from build123d import *

# Parameters (mm, degrees)
ESBO_O1_R                = 0.5
RESSALTO_EXTRUS_O1_DEPTH = 5


with BuildPart() as part:
    # Esboço1 → Ressalto-extrusão1 (new body)
    with BuildSketch(Plane.XZ.offset(5)):
        with BuildLine():
            ThreePointArc((0.88816946, -1.287165167), (0.853822869, -1.148958648), (0.919306865, -1.022496889))
            ThreePointArc((0.919306865, -1.022496889), (0.972271824, -0.972271824), (1.022496889, -0.919306865))
            ThreePointArc((1.022496889, -0.919306865), (1.148958648, -0.853822869), (1.287165167, -0.88816946))
            add(Edge.make_bspline(
                [(1.287165167, -0.88816946), (1.383791359, -0.954882813), (1.556408334, -1.073982269), (1.549215881, -1.068804746), (1.613247697, -1.099886307), (1.689593731, -1.118505632), (1.818337157, -1.137704346), (2.003981613, -1.135749512), (2.169907523, -1.103671613), (2.254570833, -1.080236252)],
                knots=[0.030903034, 0.030903034, 0.030903034, 0.030903034, 0.091208758, 0.151514483, 0.272125931, 0.39273738, 0.513348828, 0.754571725, 0.995794622, 0.995794622, 0.995794622, 0.995794622], degree=3))
            ThreePointArc((2.254570833, -1.080236252), (2.309698831, -0.956708581), (2.358064704, -0.830379945))
            add(Edge.make_bspline(
                [(1.538193866, -0.28213257), (1.653692366, -0.303284141), (1.859967032, -0.341126742), (1.851220139, -0.339701972), (1.918475453, -0.36300132), (1.985626101, -0.403820267), (2.090236992, -0.481280077), (2.220125169, -0.613932807), (2.314770006, -0.753942643), (2.358064704, -0.830379945)],
                knots=[0.030903034, 0.030903034, 0.030903034, 0.030903034, 0.091208758, 0.151514483, 0.272125931, 0.39273738, 0.513348828, 0.754571725, 0.995794622, 0.995794622, 0.995794622, 0.995794622], degree=3))
            ThreePointArc((1.538193866, -0.28213257), (1.416180392, -0.208692511), (1.373062602, -0.072966366))
            ThreePointArc((1.373062602, -0.072966366), (1.375, 0), (1.373062602, 0.072966366))
            ThreePointArc((1.373062602, 0.072966366), (1.416180392, 0.208692511), (1.538193866, 0.28213257))
            add(Edge.make_bspline(
                [(1.538193866, 0.28213257), (1.653692366, 0.303284141), (1.859967032, 0.341126742), (1.851220139, 0.339701972), (1.918475453, 0.36300132), (1.985626101, 0.403820267), (2.090236992, 0.481280077), (2.220125169, 0.613932807), (2.314770006, 0.753942643), (2.358064704, 0.830379945)],
                knots=[0.030903034, 0.030903034, 0.030903034, 0.030903034, 0.091208758, 0.151514483, 0.272125931, 0.39273738, 0.513348828, 0.754571725, 0.995794622, 0.995794622, 0.995794622, 0.995794622], degree=3))
            ThreePointArc((2.358064704, 0.830379945), (2.309698831, 0.956708581), (2.254570833, 1.080236252))
            add(Edge.make_bspline(
                [(1.287165167, 0.88816946), (1.383791359, 0.954882813), (1.556408334, 1.073982269), (1.549215881, 1.068804746), (1.613247697, 1.099886307), (1.689593731, 1.118505632), (1.818337157, 1.137704346), (2.003981613, 1.135749512), (2.169907523, 1.103671613), (2.254570833, 1.080236252)],
                knots=[0.030903034, 0.030903034, 0.030903034, 0.030903034, 0.091208758, 0.151514483, 0.272125931, 0.39273738, 0.513348828, 0.754571725, 0.995794622, 0.995794622, 0.995794622, 0.995794622], degree=3))
            ThreePointArc((1.287165167, 0.88816946), (1.148958648, 0.853822869), (1.022496889, 0.919306865))
            ThreePointArc((1.022496889, 0.919306865), (0.972271824, 0.972271824), (0.919306865, 1.022496889))
            ThreePointArc((0.919306865, 1.022496889), (0.853822869, 1.148958648), (0.88816946, 1.287165167))
            add(Edge.make_bspline(
                [(0.88816946, 1.287165167), (0.954882813, 1.383791359), (1.073982269, 1.556408334), (1.068804746, 1.549215881), (1.099886307, 1.613247697), (1.118505632, 1.689593731), (1.137704346, 1.818337157), (1.135749512, 2.003981613), (1.103671613, 2.169907523), (1.080236252, 2.254570833)],
                knots=[0.030903034, 0.030903034, 0.030903034, 0.030903034, 0.091208758, 0.151514483, 0.272125931, 0.39273738, 0.513348828, 0.754571725, 0.995794622, 0.995794622, 0.995794622, 0.995794622], degree=3))
            ThreePointArc((1.080236252, 2.254570833), (0.956708581, 2.309698831), (0.830379945, 2.358064704))
            add(Edge.make_bspline(
                [(0.28213257, 1.538193866), (0.303284141, 1.653692366), (0.341126742, 1.859967032), (0.339701972, 1.851220139), (0.36300132, 1.918475453), (0.403820267, 1.985626101), (0.481280077, 2.090236992), (0.613932807, 2.220125169), (0.753942643, 2.314770006), (0.830379945, 2.358064704)],
                knots=[0.030903034, 0.030903034, 0.030903034, 0.030903034, 0.091208758, 0.151514483, 0.272125931, 0.39273738, 0.513348828, 0.754571725, 0.995794622, 0.995794622, 0.995794622, 0.995794622], degree=3))
            ThreePointArc((0.28213257, 1.538193866), (0.208692511, 1.416180392), (0.072966366, 1.373062602))
            ThreePointArc((0.072966366, 1.373062602), (0, 1.375), (-0.072966366, 1.373062602))
            ThreePointArc((-0.072966366, 1.373062602), (-0.208692511, 1.416180392), (-0.28213257, 1.538193866))
            add(Edge.make_bspline(
                [(-0.28213257, 1.538193866), (-0.303284141, 1.653692366), (-0.341126742, 1.859967032), (-0.339701972, 1.851220139), (-0.36300132, 1.918475453), (-0.403820267, 1.985626101), (-0.481280077, 2.090236992), (-0.613932807, 2.220125169), (-0.753942643, 2.314770006), (-0.830379945, 2.358064704)],
                knots=[0.030903034, 0.030903034, 0.030903034, 0.030903034, 0.091208758, 0.151514483, 0.272125931, 0.39273738, 0.513348828, 0.754571725, 0.995794622, 0.995794622, 0.995794622, 0.995794622], degree=3))
            ThreePointArc((-0.830379945, 2.358064704), (-0.956708581, 2.309698831), (-1.080236252, 2.254570833))
            add(Edge.make_bspline(
                [(-0.88816946, 1.287165167), (-0.954882813, 1.383791359), (-1.073982269, 1.556408334), (-1.068804746, 1.549215881), (-1.099886307, 1.613247697), (-1.118505632, 1.689593731), (-1.137704346, 1.818337157), (-1.135749512, 2.003981613), (-1.103671613, 2.169907523), (-1.080236252, 2.254570833)],
                knots=[0.030903034, 0.030903034, 0.030903034, 0.030903034, 0.091208758, 0.151514483, 0.272125931, 0.39273738, 0.513348828, 0.754571725, 0.995794622, 0.995794622, 0.995794622, 0.995794622], degree=3))
            ThreePointArc((-0.88816946, 1.287165167), (-0.853822869, 1.148958648), (-0.919306865, 1.022496889))
            ThreePointArc((-0.919306865, 1.022496889), (-0.972271824, 0.972271824), (-1.022496889, 0.919306865))
            ThreePointArc((-1.022496889, 0.919306865), (-1.148958648, 0.853822869), (-1.287165167, 0.88816946))
            add(Edge.make_bspline(
                [(-1.287165167, 0.88816946), (-1.383791359, 0.954882813), (-1.556408334, 1.073982269), (-1.549215881, 1.068804746), (-1.613247697, 1.099886307), (-1.689593731, 1.118505632), (-1.818337157, 1.137704346), (-2.003981613, 1.135749512), (-2.169907523, 1.103671613), (-2.254570833, 1.080236252)],
                knots=[0.030903034, 0.030903034, 0.030903034, 0.030903034, 0.091208758, 0.151514483, 0.272125931, 0.39273738, 0.513348828, 0.754571725, 0.995794622, 0.995794622, 0.995794622, 0.995794622], degree=3))
            ThreePointArc((-2.254570833, 1.080236252), (-2.309698831, 0.956708581), (-2.358064704, 0.830379945))
            add(Edge.make_bspline(
                [(-1.538193866, 0.28213257), (-1.653692366, 0.303284141), (-1.859967032, 0.341126742), (-1.851220139, 0.339701972), (-1.918475453, 0.36300132), (-1.985626101, 0.403820267), (-2.090236992, 0.481280077), (-2.220125169, 0.613932807), (-2.314770006, 0.753942643), (-2.358064704, 0.830379945)],
                knots=[0.030903034, 0.030903034, 0.030903034, 0.030903034, 0.091208758, 0.151514483, 0.272125931, 0.39273738, 0.513348828, 0.754571725, 0.995794622, 0.995794622, 0.995794622, 0.995794622], degree=3))
            ThreePointArc((-1.538193866, 0.28213257), (-1.416180392, 0.208692511), (-1.373062602, 0.072966366))
            ThreePointArc((-1.373062602, 0.072966366), (-1.375, 0), (-1.373062602, -0.072966366))
            ThreePointArc((-1.373062602, -0.072966366), (-1.416180392, -0.208692511), (-1.538193866, -0.28213257))
            add(Edge.make_bspline(
                [(-1.538193866, -0.28213257), (-1.653692366, -0.303284141), (-1.859967032, -0.341126742), (-1.851220139, -0.339701972), (-1.918475453, -0.36300132), (-1.985626101, -0.403820267), (-2.090236992, -0.481280077), (-2.220125169, -0.613932807), (-2.314770006, -0.753942643), (-2.358064704, -0.830379945)],
                knots=[0.030903034, 0.030903034, 0.030903034, 0.030903034, 0.091208758, 0.151514483, 0.272125931, 0.39273738, 0.513348828, 0.754571725, 0.995794622, 0.995794622, 0.995794622, 0.995794622], degree=3))
            ThreePointArc((-2.358064704, -0.830379945), (-2.309698831, -0.956708581), (-2.254570833, -1.080236252))
            add(Edge.make_bspline(
                [(-1.287165167, -0.88816946), (-1.383791359, -0.954882813), (-1.556408334, -1.073982269), (-1.549215881, -1.068804746), (-1.613247697, -1.099886307), (-1.689593731, -1.118505632), (-1.818337157, -1.137704346), (-2.003981613, -1.135749512), (-2.169907523, -1.103671613), (-2.254570833, -1.080236252)],
                knots=[0.030903034, 0.030903034, 0.030903034, 0.030903034, 0.091208758, 0.151514483, 0.272125931, 0.39273738, 0.513348828, 0.754571725, 0.995794622, 0.995794622, 0.995794622, 0.995794622], degree=3))
            ThreePointArc((-1.287165167, -0.88816946), (-1.148958648, -0.853822869), (-1.022496889, -0.919306865))
            ThreePointArc((-1.022496889, -0.919306865), (-0.972271824, -0.972271824), (-0.919306865, -1.022496889))
            ThreePointArc((-0.919306865, -1.022496889), (-0.853822869, -1.148958648), (-0.88816946, -1.287165167))
            add(Edge.make_bspline(
                [(-0.88816946, -1.287165167), (-0.954882813, -1.383791359), (-1.073982269, -1.556408334), (-1.068804746, -1.549215881), (-1.099886307, -1.613247697), (-1.118505632, -1.689593731), (-1.137704346, -1.818337157), (-1.135749512, -2.003981613), (-1.103671613, -2.169907523), (-1.080236252, -2.254570833)],
                knots=[0.030903034, 0.030903034, 0.030903034, 0.030903034, 0.091208758, 0.151514483, 0.272125931, 0.39273738, 0.513348828, 0.754571725, 0.995794622, 0.995794622, 0.995794622, 0.995794622], degree=3))
            ThreePointArc((-1.080236252, -2.254570833), (-0.956708581, -2.309698831), (-0.830379945, -2.358064704))
            add(Edge.make_bspline(
                [(-0.28213257, -1.538193866), (-0.303284141, -1.653692366), (-0.341126742, -1.859967032), (-0.339701972, -1.851220139), (-0.36300132, -1.918475453), (-0.403820267, -1.985626101), (-0.481280077, -2.090236992), (-0.613932807, -2.220125169), (-0.753942643, -2.314770006), (-0.830379945, -2.358064704)],
                knots=[0.030903034, 0.030903034, 0.030903034, 0.030903034, 0.091208758, 0.151514483, 0.272125931, 0.39273738, 0.513348828, 0.754571725, 0.995794622, 0.995794622, 0.995794622, 0.995794622], degree=3))
            ThreePointArc((-0.28213257, -1.538193866), (-0.208692511, -1.416180392), (-0.072966366, -1.373062602))
            ThreePointArc((-0.072966366, -1.373062602), (0, -1.375), (0.072966366, -1.373062602))
            ThreePointArc((0.072966366, -1.373062602), (0.208692511, -1.416180392), (0.28213257, -1.538193866))
            add(Edge.make_bspline(
                [(0.28213257, -1.538193866), (0.303284141, -1.653692366), (0.341126742, -1.859967032), (0.339701972, -1.851220139), (0.36300132, -1.918475453), (0.403820267, -1.985626101), (0.481280077, -2.090236992), (0.613932807, -2.220125169), (0.753942643, -2.314770006), (0.830379945, -2.358064704)],
                knots=[0.030903034, 0.030903034, 0.030903034, 0.030903034, 0.091208758, 0.151514483, 0.272125931, 0.39273738, 0.513348828, 0.754571725, 0.995794622, 0.995794622, 0.995794622, 0.995794622], degree=3))
            ThreePointArc((0.830379945, -2.358064704), (0.956708581, -2.309698831), (1.080236252, -2.254570833))
            add(Edge.make_bspline(
                [(0.88816946, -1.287165167), (0.954882813, -1.383791359), (1.073982269, -1.556408334), (1.068804746, -1.549215881), (1.099886307, -1.613247697), (1.118505632, -1.689593731), (1.137704346, -1.818337157), (1.135749512, -2.003981613), (1.103671613, -2.169907523), (1.080236252, -2.254570833)],
                knots=[0.030903034, 0.030903034, 0.030903034, 0.030903034, 0.091208758, 0.151514483, 0.272125931, 0.39273738, 0.513348828, 0.754571725, 0.995794622, 0.995794622, 0.995794622, 0.995794622], degree=3))
        make_face()
        with Locations(Location((0, 0, 0), (0, 0, 90))):
            Circle(ESBO_O1_R, mode=Mode.SUBTRACT)
    extrude(amount=-RESSALTO_EXTRUS_O1_DEPTH)


solid = part.part
The model under review builds one solid part; all positions refer to its coordinate system, in mm. Give positions to 0.01 mm unless a question says otherwise; leave off trailing zeros. Write each loop counter-clockwise with the first axis right and the second up, starting at its lowest first coordinate (ties: lowest second). Pieces come first, ordered by that corner, then holes.
1. For P1, Ø1, axis at y = -4.5, z = 2, coming from the -X side; P2, Ø2, axis at y = -4, z = -1.5, coming from the +X side, all flat-tipped, find the tip position at first contact; note any pin that passes through.
2. Add section B-B, the plane x = 0. Write out the cut boundary in (y, z) (3 decimals).
3. Wall thickness on L1, parallel to X at y = -1.7, z = -0.05; L2, parallel to X at y = -4, z = 1.75; L3, parallel to Z at x = 1.65, y = -2.9: over which ranges is each line inside the solid? List them lowest first.
4. Add section A-A, the plane z = 0. Write out the cut boundary in (x, y) (3 decimals).
5. Draft analysis for pull direction Z (two halves, no side actions). For faces 1 (the cylindrical face through (0.488, -2.535, -0.108)), 2 (the flat face through (-1, 0, 0)), state which applies: +Z half, -Z half, draft (parallel to the pull), parting line (faces both ways), or undercut.
Worked answers:
1. P1: stops at x = -1.14
1. P2: stops at x = 2.36
2. outline: (-5, -1.375) - (0, -1.375) - (0, -0.5) - (-5, -0.5) - close; (-5, 0.5) - (0, 0.5) - (0, 1.375) - (-5, 1.375) - close
3. L1: x = -1.37 to -0.5, 0.5 to 1.37
3. L2: x = -1.13 to -0.32, 0.32 to 1.13
3. L3: z = -1.11 to -0.3, 0.3 to 1.11
4. outline: (-1.375, -5) - (-0.5, -5) - (-0.5, 0) - (-1.375, 0) - close; (0.5, -5) - (1.375, -5) - (1.375, 0) - (0.5, 0) - close
5. face 1: undercut
5. face 2: draft
